from build123d import *

# Parameters (mm, degrees)
SKETCH1_W           = 27.6
SKETCH1_H           = 26.6
BOSS_EXTRUDE1_DEPTH = 2
BOSS_EXTRUDE1_TAPER = 30
SKETCH2_W           = 5.514509834
SKETCH2_H           = 2
BOSS_EXTRUDE2_DEPTH = 13.3
SKETCH3_R           = 1.27
CUT_EXTRUDE1_DEPTH  = 3.0000001
FILLET5_R           = 1


with BuildPart() as part:
    # Sketch1 → Boss-Extrude1 (new body)
    with BuildSketch(Plane(origin=(0, 0, 0), x_dir=(1, 0, 0), z_dir=(0, 1, 0))):
        Rectangle(SKETCH1_W, SKETCH1_H)
    extrude(amount=BOSS_EXTRUDE1_DEPTH, taper=BOSS_EXTRUDE1_TAPER)

    # Sketch2 → Boss-Extrude2 (add)
    with BuildSketch(Plane.XY):
        with Locations((0, 1)):
            Rectangle(SKETCH2_W, SKETCH2_H)
    extrude(amount=BOSS_EXTRUDE2_DEPTH)

    # Sketch3 → Cut-Extrude1 (cut, through all)
    with BuildSketch(Plane(origin=(0, 0, 0), x_dir=(1, 0, 0), z_dir=(0, 1, 0))):
        with Locations((-9.87, -10.07)):
            Circle(SKETCH3_R)
    extrude(amount=CUT_EXTRUDE1_DEPTH, mode=Mode.SUBTRACT)

    # Fillet5
    fillet5_edges = [part.edges().sort_by_distance(p)[0] for p in [
        (-12.645299462, 2, 0),
        (-7.701277189, 2, 12.145299462),
        (7.701277189, 2, 12.145299462),
        (12.645299462, 2, 0),
        (0, 2, -12.145299462),
    ]]
    fillet(fillet5_edges, radius=FILLET5_R)


solid = part.part
Geometry check sheet. Reference: the model listing, model coordinates, mm. A direction names the side the tool comes from. Give positions to 0.01 mm unless a question says otherwise; leave off trailing zeros. Use a Markdown table: item, result.
Item 1: Depth check by flat-ended pin: P1, Ø3, axis at x = -9.87, z = 10.07, coming from the -Y side; P2, Ø1, axis at x = -7.5, y = 1, coming from the -Z side. Enter the tip coordinate at first touch or a pass-through.
Answers follow:
| item | result |
|---|---|
| P1 | stops at y = 0 |
| P2 | stops at z = -13.01 |
Item 2: Material ranges on line 1 along X through (y, z) = (0.7, 10.07); line 2 along X through (y, z) = (1.05, 10.07); line 3 along Z through (x, y) = (-9.87, 0.65), recorded low to high.
Answers follow:
| item | result |
|---|---|
| line 1 | x = -13.4 to -11.14, -8.6 to 13.4 |
| line 2 | x = -13.19 to -11.14, -8.6 to 13.19 |
| line 3 | z = -12.92 to 8.8, 11.34 to 12.92 |
Item 3: Draft check along Z on faces 1 (the flat face through (2.757, 1, 13)), 2 (the cylindrical face through (-9.284, 0.986, 11.197)), 3 (the flat face through (0, 1, 13.3)). Enter one of: +Z half, -Z half, draft (parallel to the pull), parting line (faces both ways), or undercut.
Answers follow:
| item | result |
|---|---|
| face 1 | draft |
| face 2 | undercut |
| face 3 | +Z half |
Item 4: Tool access check on faces 4 (the flat face through (0, 0, 0)), 5 (the flat face through (-2.757, 1, 13)). Record the directions out of +Z, -Z, +X, -X, +Y, -Y that give a thin tool (end or side, any length) a straight path to the whole face; none if there is none.
Answers follow:
| item | result |
|---|---|
| face 4 | +Z, -Z, +X, -X, -Y |
| face 5 | +Z, -X, +Y |
